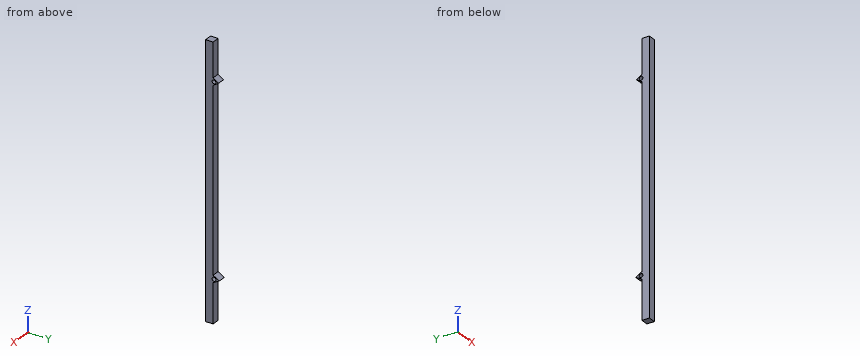
```python
from build123d import *

# Parameters (mm, degrees)
SKETCH1_R           = 1.25
BOSS_EXTRUDE1_DEPTH = 5


with BuildPart() as part:
    # Sketch1 → Boss-Extrude1 (new body)
    with BuildSketch(Plane(origin=(0, 0, 0), x_dir=(0, 0, -1), z_dir=(1, 0, 0))):
        Polygon((25.233, 8.638537032), (22.869893181, 5), (0, 5), (0, 0), (180, 0), (180, 5), (153.59702619, 5), (151.233, 9.21189857), (148.866471386, 5), (27.622231329, 5), align=None)
        with Locations((25.233, 5.593756264)):
            Circle(SKETCH1_R, mode=Mode.SUBTRACT)
        with Locations((151.233, 5.593756264)):
            Circle(SKETCH1_R, mode=Mode.SUBTRACT)
    extrude(amount=-BOSS_EXTRUDE1_DEPTH)


solid = part.part
```
Geometry check sheet. Reference: the model listing, model coordinates, mm. Give positions to 0.01 mm unless a question says otherwise; leave off trailing zeros. Loops run counter-clockwise (first coordinate to the right, second up) from the corner with the lowest first, then second, coordinate; pieces in that order, holes last. Notation, with made-up numbers: (-24, -17) - (22, -17) arc R22 cw to (22, 15) - close; hole circle Ø1 at (-31.5, 31). An arc over 180 degrees is marked (long way). Use CSV: the item, a comma, the result in double quotes. Start each with the question number.
Q1. Section check B-B, the plane z = -72.5. Record the cut outline in (x, y), and give its area (3 significant figures).
Q2. Scan lines: probe 1 along Z at (x, y) = (-2.7, 6.5); probe 2 along Y at (x, z) = (-1.9, -72); probe 3 along Z at (x, y) = (-4.15, 7.5). Record each from-to range of solid material in increasing order. Write a range as from..to.
Q3. Go/stop test with a flat-tipped pin: pin 1 Ø2.5 at (x, z) = (-2, -78.5) entering from +Y. Record where the tip stops, or that it passes through.
Q4. Section check A-A, the plane x = -3.2. Record the cut outline in (y, z), and give its area (3 significant figures).
Findings below:
1,outline,"(-5, 0) - (0, 0) - (0, 5) - (-5, 5) - close"
1,area,"25.0 mm^2"
2,probe 1,"z = -152.76..-152.09, -150.37..-149.71, -26.64..-26.09, -24.37..-23.84"
2,probe 2,"y = 0..5"
2,probe 3,"z = -152.19..-150.27, -25.98..-24.49"
3,pin 1,"stops at y = 5"
4,outline,"(0, -180) - (5, -180) - (5, -153.6) - (9.21, -151.23) - (5, -148.87) - (5, -27.62) - (8.64, -25.23) - (5, -22.87) - (5, 0) - (0, 0) - close; hole circle Ø2.5 at (5.59, -151.23); hole circle Ø2.5 at (5.59, -25.23)"
4,area,"909 mm^2"
